CAD build for the part. Positions are in the model's coordinates, mm. Coordinates: 2 decimals unless noted, no trailing zeros. Write each loop counter-clockwise with the first axis right and the second up, starting at its lowest first coordinate (ties: lowest second). Pieces come first, ordered by that corner, then holes. Notation, with made-up numbers: M 41.5,53.25 L 81.5,53.25 A32 cw 81.5,80.25 Z; hole C 44,38 d11. An arc over 180 degrees is marked long. Put each result on its own line as item: value. Start each with the question number.
```python
from build123d import *

# Parameters (mm, degrees)
SKETCH1_R           = 76
SKETCH1_R_2         = 27.051
SKETCH1_R_3         = 2
BOSS_EXTRUDE1_DEPTH = 7
SKETCH4_R           = 6.25
CUT_EXTRUDE1_DEPTH  = 10
FILLET1_R           = 5


with BuildPart() as part:
    # Sketch1 → Boss-Extrude1 (new body)
    with BuildSketch(Plane(origin=(0, 0, 0), x_dir=(1, 0, 0), z_dir=(0, 1, 0))):
        with Locations(Location((0, 0, 0), (0, 0, 270))):
            Circle(SKETCH1_R)
        with Locations(Location((0, 0, 0), (0, 0, 270))):
            Circle(SKETCH1_R_2, mode=Mode.SUBTRACT)
        with Locations(Location((0, 62.5, 0), (0, 0, 270))):
            Circle(SKETCH1_R_3, mode=Mode.SUBTRACT)
        with Locations(Location((62.5, 0, 0), (0, 0, 270))):
            Circle(SKETCH1_R_3, mode=Mode.SUBTRACT)
        with Locations(Location((0, -62.5, 0), (0, 0, 270))):
            Circle(SKETCH1_R_3, mode=Mode.SUBTRACT)
        with Locations(Location((-62.5, 0, 0), (0, 0, 270))):
            Circle(SKETCH1_R_3, mode=Mode.SUBTRACT)
    extrude(amount=BOSS_EXTRUDE1_DEPTH)

    # Sketch4 → Cut-Extrude1 (cut)
    with BuildSketch(Plane(origin=(0, 7, 0), x_dir=(1, 0, 0), z_dir=(0, 1, 0))):
        with BuildLine():
            Line((27.751246841, -43.661149418), (17.007161012, -32.917063589))
            ThreePointArc((17.007161012, -32.917063589), (15.274204293, -33.756114768), (13.5, -34.504008477))
            Line((13.5, -34.504008477), (13.5, -62.5))
            ThreePointArc((13.5, -62.5), (25.524772494, -58.625813335), (36.553123822, -52.463026398))
            Line((36.553123822, -52.463026398), (27.751246841, -43.661149418))
        make_face()
        with BuildLine():
            Line((62.5, -13.5), (34.504008477, -13.5))
            ThreePointArc((34.504008477, -13.5), (33.756114768, -15.274204293), (32.917063589, -17.007161012))
            Line((32.917063589, -17.007161012), (43.66114941, -27.751246833))
            Line((43.66114941, -27.751246833), (52.463026398, -36.553123822))
            ThreePointArc((52.463026398, -36.553123822), (58.625813335, -25.524772494), (62.5, -13.5))
        make_face()
        with BuildLine():
            ThreePointArc((-13.5, -34.504008477), (-15.274204293, -33.756114768), (-17.007161012, -32.917063589))
            Line((-17.007161012, -32.917063589), (-27.751246874, -43.66114945))
            Line((-27.751246874, -43.66114945), (-36.553123822, -52.463026398))
            ThreePointArc((-36.553123822, -52.463026398), (-25.524772494, -58.625813335), (-13.5, -62.5))
            Line((-13.5, -62.5), (-13.5, -34.504008477))
        make_face()
        with BuildLine():
            ThreePointArc((-32.917063589, -17.007161012), (-33.756114768, -15.274204293), (-34.504008477, -13.5))
            Line((-34.504008477, -13.5), (-62.5, -13.5))
            ThreePointArc((-62.5, -13.5), (-58.625813335, -25.524772494), (-52.463026398, -36.553123822))
            Line((-52.463026398, -36.553123822), (-43.661149471, -27.751246894))
            Line((-43.661149471, -27.751246894), (-32.917063589, -17.007161012))
        make_face()
        with BuildLine():
            ThreePointArc((-34.504008477, 13.5), (-33.756114768, 15.274204293), (-32.917063589, 17.007161012))
            Line((-32.917063589, 17.007161012), (-43.66114943, 27.751246854))
            Line((-43.66114943, 27.751246854), (-52.463026398, 36.553123822))
            ThreePointArc((-52.463026398, 36.553123822), (-58.625813335, 25.524772494), (-62.5, 13.5))
            Line((-62.5, 13.5), (-34.504008477, 13.5))
        make_face()
        with BuildLine():
            ThreePointArc((-17.007161012, 32.917063589), (-15.274204293, 33.756114768), (-13.5, 34.504008477))
            Line((-13.5, 34.504008477), (-13.5, 62.5))
            ThreePointArc((-13.5, 62.5), (-25.524772494, 58.625813335), (-36.553123822, 52.463026398))
            Line((-36.553123822, 52.463026398), (-27.751246874, 43.66114945))
            Line((-27.751246874, 43.66114945), (-17.007161012, 32.917063589))
        make_face()
        with BuildLine():
            ThreePointArc((36.553123822, 52.463026398), (25.524772494, 58.625813335), (13.5, 62.5))
            Line((13.5, 62.5), (13.5, 34.504008477))
            ThreePointArc((13.5, 34.504008477), (15.274204293, 33.756114768), (17.007161012, 32.917063589))
            Line((17.007161012, 32.917063589), (27.751246906, 43.661149483))
            Line((27.751246906, 43.661149483), (36.553123822, 52.463026398))
        make_face()
        with BuildLine():
            ThreePointArc((62.5, 13.5), (58.625813335, 25.524772494), (52.463026398, 36.553123822))
            Line((52.463026398, 36.553123822), (43.66114945, 27.751246874))
            Line((43.66114945, 27.751246874), (32.917063589, 17.007161012))
            ThreePointArc((32.917063589, 17.007161012), (33.756114768, 15.274204293), (34.504008477, 13.5))
            Line((34.504008477, 13.5), (62.5, 13.5))
        make_face()
        with Locations(Location((35.706198162, 35.706198162, 0), (0, 0, 270))):
            Circle(SKETCH4_R)
        with Locations(Location((35.706198162, -35.706198162, 0), (0, 0, 270))):
            Circle(SKETCH4_R)
        with Locations(Location((-35.706198162, -35.706198162, 0), (0, 0, 270))):
            Circle(SKETCH4_R)
        with Locations(Location((-35.706198162, 35.706198162, 0), (0, 0, 270))):
            Circle(SKETCH4_R)
    extrude(amount=-CUT_EXTRUDE1_DEPTH, mode=Mode.SUBTRACT)

    # Fillet1
    # the kernel refuses this fillet: 5 mm, written as the material it adds along each edge
    with BuildSketch(Plane(origin=(34.504008477, 7, 13.5), x_dir=(1, 0, 0), z_dir=(0, -1, 0)), Plane(origin=(13.5, 7, -34.504008477), x_dir=(0, 0, -1), z_dir=(0, -1, 0)), Plane(origin=(-34.504008477, 7, -13.5), x_dir=(-1, 0, 0), z_dir=(0, -1, 0)), Plane(origin=(-13.5, 7, 34.504008477), x_dir=(0, 0, 1), z_dir=(0, -1, 0))) as fillet1_piece_1:
        with BuildLine():
            CenterArc((3.258891319, 5), FILLET1_R, 206.100178987, 63.899821013)
            ThreePointArc((-1.231239688, 2.800290124), (-0.586707725, 1.412857227), (0, 0))
            Line((0, 0), (3.258891319, 0))
        make_face()
    extrude(amount=7)
    with BuildSketch(Plane(origin=(62.5, 7, 13.5), x_dir=(-1, 0, 0), z_dir=(0, -1, 0))) as fillet1_piece_2:
        with BuildLine():
            CenterArc((6.537189081, -5), FILLET1_R, 90, 108.2926811)
            ThreePointArc((1.789861186, -6.569355874), (0.807426008, -3.308519097), (0, 0))
            Line((0, 0), (6.537189081, 0))
        make_face()
    extrude(amount=7)
    with BuildSketch(Plane(origin=(52.463026398, 7, 36.553123822), x_dir=(-0.7071067811865521, 0, -0.707106781186543), z_dir=(0, -1, 0)), Plane(origin=(-36.553123822, 7, 52.463026398), x_dir=(0.7071067811865515, 0, -0.7071067811865436), z_dir=(0, -1, 0))) as fillet1_piece_3:
        with BuildLine():
            CenterArc((6.286852353, 5), FILLET1_R, 163.996405934, 106.003594066)
            ThreePointArc((1.480630334, 6.378488268), (0.658610883, 3.208210045), (0, 0))
            Line((0, 0), (6.286852353, 0))
        make_face()
    extrude(amount=7)
    with BuildSketch(Plane(origin=(32.917063589, 7, 17.007161012), x_dir=(0.4193809358930841, 0, -0.907810349472532), z_dir=(0, -1, 0)), Plane(origin=(17.007161012, 7, -32.917063589), x_dir=(-0.9078103494725283, 0, -0.41938093589309267), z_dir=(0, -1, 0)), Plane(origin=(-32.917063589, 7, -17.007161012), x_dir=(-0.4193809358930852, 0, 0.9078103494725317), z_dir=(0, -1, 0))) as fillet1_piece_4:
        with BuildLine():
            CenterArc((3.489548398, 4.995132399), FILLET1_R, 200.204490443, 67.267112024)
            Line((-1.202781391, 3.268273647), (0, 0))
            ThreePointArc((0, 0), (1.634487847, 0.036069898), (3.268975694, 0))
        make_face()
    extrude(amount=7)
    with BuildSketch(Plane(origin=(32.917063589, 7, -17.007161012), x_dir=(0.7071067811865526, 0, -0.7071067811865425), z_dir=(0, -1, 0)), Plane(origin=(-17.007161012, 7, -32.917063589), x_dir=(-0.7071067811865506, 0, -0.7071067811865445), z_dir=(0, -1, 0)), Plane(origin=(-32.917063589, 7, 17.007161012), x_dir=(-0.7071067811865506, 0, 0.7071067811865445), z_dir=(0, -1, 0)), Plane(origin=(17.007161012, 7, 32.917063589), x_dir=(0.7071067811865501, 0, 0.707106781186545), z_dir=(0, -1, 0))) as fillet1_piece_5:
        with BuildLine():
            CenterArc((3.482570273, 5), FILLET1_R, 202.732887976, 67.267112024)
            ThreePointArc((-1.129011858, 3.067822406), (-0.530655558, 1.546368727), (0, 0))
            Line((0, 0), (3.482570273, 0))
        make_face()
    extrude(amount=7)
    with BuildSketch(Plane(origin=(34.504008477, 7, -13.5), x_dir=(1, 0, 0), z_dir=(0, -1, 0))) as fillet1_piece_6:
        with BuildLine():
            CenterArc((3.258891319, -5), FILLET1_R, 90, 63.899821013)
            ThreePointArc((-1.231239688, -2.800290124), (-0.586707725, -1.412857227), (0, 0))
            Line((0, 0), (3.258891319, 0))
        make_face()
    extrude(amount=7)
    with BuildSketch(Plane(origin=(62.5, 7, -13.5), x_dir=(-1, 0, 0), z_dir=(0, -1, 0)), Plane(origin=(-13.5, 7, -62.5), x_dir=(0, 0, 1), z_dir=(0, -1, 0)), Plane(origin=(-62.5, 7, 13.5), x_dir=(1, 0, 0), z_dir=(0, -1, 0)), Plane(origin=(13.5, 7, 62.5), x_dir=(0, 0, -1), z_dir=(0, -1, 0))) as fillet1_piece_7:
        with BuildLine():
            CenterArc((6.537189081, 5), FILLET1_R, 161.7073189, 108.2926811)
            ThreePointArc((1.789861186, 6.569355874), (0.807426008, 3.308519097), (0, 0))
            Line((0, 0), (6.537189081, 0))
        make_face()
    extrude(amount=7)
    with BuildSketch(Plane(origin=(52.463026398, 7, -36.553123822), x_dir=(0.5289042688396526, 0, 0.848681491728901), z_dir=(0, -1, 0))) as fillet1_piece_8:
        with BuildLine():
            CenterArc((6.292063112, 4.993441128), FILLET1_R, 166.931450544, 106.003594066)
            Line((1.421561948, 6.124024341), (0, 0))
            ThreePointArc((0, 0), (3.274041034, -0.08387667), (6.548082068, 0))
        make_face()
    extrude(amount=7)
    with BuildSketch(Plane(origin=(36.553123822, 7, -52.463026398), x_dir=(-0.8486814917288963, 0, -0.52890426883966), z_dir=(0, -1, 0)), Plane(origin=(-52.463026398, 7, -36.553123822), x_dir=(-0.5289042688396536, 0, 0.8486814917289003), z_dir=(0, -1, 0))) as fillet1_piece_9:
        with BuildLine():
            CenterArc((6.292063112, -4.993441128), FILLET1_R, 87.06495539, 106.003594066)
            Line((1.421561948, -6.124024341), (0, 0))
            ThreePointArc((0, 0), (3.274041034, 0.08387667), (6.548082068, 0))
        make_face()
    extrude(amount=7)
    with BuildSketch(Plane(origin=(13.5, 7, -62.5), x_dir=(0.9648302017860143, 0, 0.26287388938720957), z_dir=(0, -1, 0)), Plane(origin=(-62.5, 7, -13.5), x_dir=(0.2628738893872084, 0, -0.9648302017860146), z_dir=(0, -1, 0)), Plane(origin=(-13.5, 7, 62.5), x_dir=(-0.9648302017860145, 0, -0.26287388938720885), z_dir=(0, -1, 0))) as fillet1_piece_10:
        with BuildLine():
            CenterArc((6.542607328, 4.992908013), FILLET1_R, 164.759342849, 108.2926811)
            Line((1.718456319, 6.30727746), (0, 0))
            ThreePointArc((0, 0), (3.404410363, -0.090694285), (6.808820725, 0))
        make_face()
    extrude(amount=7)
    with BuildSketch(Plane(origin=(-36.553123822, 7, -52.463026398), x_dir=(0.707106781186552, 0, 0.7071067811865429), z_dir=(0, -1, 0)), Plane(origin=(-52.463026398, 7, 36.553123822), x_dir=(0.7071067811865515, 0, -0.7071067811865436), z_dir=(0, -1, 0)), Plane(origin=(36.553123822, 7, 52.463026398), x_dir=(-0.7071067811865527, 0, -0.7071067811865425), z_dir=(0, -1, 0))) as fillet1_piece_11:
        with BuildLine():
            CenterArc((6.286852353, -5), FILLET1_R, 90, 106.003594066)
            ThreePointArc((1.480630334, -6.378488268), (0.658610883, -3.208210045), (0, 0))
            Line((0, 0), (6.286852353, 0))
        make_face()
    extrude(amount=7)
    with BuildSketch(Plane(origin=(-13.5, 7, -34.504008477), x_dir=(-0.9154220062230544, 0, 0.4024954043496127), z_dir=(0, -1, 0)), Plane(origin=(-34.504008477, 7, 13.5), x_dir=(0.4024954043496181, 0, 0.915422006223052), z_dir=(0, -1, 0)), Plane(origin=(13.5, 7, 34.504008477), x_dir=(0.915422006223051, 0, -0.40249540434962), z_dir=(0, -1, 0))) as fillet1_piece_12:
        with BuildLine():
            CenterArc((3.265421252, 4.995737851), FILLET1_R, 203.734271223, 63.899821013)
            Line((-1.311688779, 2.983260829), (0, 0))
            ThreePointArc((0, 0), (1.52950776, 0.031583378), (3.059015519, 0))
        make_face()
    extrude(amount=7)
    with BuildSketch(Plane(origin=(-17.007161012, 7, 32.917063589), x_dir=(-0.7071067811865496, 0, 0.7071067811865455), z_dir=(0, -1, 0))) as fillet1_piece_13:
        with BuildLine():
            CenterArc((3.482570273, -5), FILLET1_R, 90, 67.267112024)
            ThreePointArc((-1.129011858, -3.067822406), (-0.530655558, -1.546368727), (0, 0))
            Line((0, 0), (3.482570273, 0))
        make_face()
    extrude(amount=7)


solid = part.part
```
(1) Two-plate mould, pull along Z, no slides. Class faces 1 (the face through (33.514, 3.549, -52.313)), 2 (the face through (22, 7, -24)), 3 (the face through (34.165, 3.549, -17.496)): +Z half, -Z half, draft (parallel to the pull), parting line (faces both ways), or undercut.
(2) Drill centre lines: line 1 (X direction, y = 3, z = 0); line 2 (X direction, y = 5.5, z = 22.5); line 3 (Z direction, x = 15.5, y = 3.75). Where is each one in solid material? Low to high. Write a range as [from, to].
(3) Drop flat-ended pins along their axis: pin 1 (7.5 mm diameter, centred on x = 35.71, z = -35.71, fed in from -Y); pin 2 (4 mm diameter, centred on y = 2.5, z = 11.5, fed in from +X); pin 3 (3 mm diameter, centred on x = 55.5, y = 4, fed in from -Z); pin 4 (1.5 mm diameter, centred on x = 57, y = 4.5, fed in from -Z). Give the stop position or say it passes through.
(4) Slice it at D-D, the plane y = 5. State how many separate pieces and enclosed holes the cut face has, then the cut area to 3 significant figures.
(5) Slice it at A-A, the plane x = 0. Write the cut outline in (y, z), then the cut area to 3 significant figures.
(6) Slice it at C-C, the plane z = -52.5. Write the cut outline in (x, y), then the cut area to 3 significant figures.
(7) Slice it at B-B, the plane z = 0. Write the cut outline in (x, y), then the cut area to 3 significant figures.
Result set:
1. face 1: undercut
1. face 2: draft
1. face 3: undercut
2. line 1: x = [-76, -64.5], [-60.5, -27.05], [27.05, 60.5], [64.5, 76]
2. line 2: x = [-72.59, -59.85], [-38.41, -15.02], [15.02, 38.41], [59.85, 72.59]
2. line 3: z = [-74.4, -59.96], [-33.93, -22.17], [22.17, 33.93], [59.96, 74.4]
3. pin 1: passes through
3. pin 2: stops at x = 75.4
3. pin 3: stops at z = -53.48
3. pin 4: stops at z = -51.11
4. separate pieces: 1
4. enclosed holes: 17
4. area: 12,300 mm^2
5. outline: M 0,-76 L 7,-76 L 7,-64.5 L 0,-64.5 Z; M 0,-60.5 L 7,-60.5 L 7,-27.05 L 0,-27.05 Z; M 0,27.05 L 7,27.05 L 7,60.5 L 0,60.5 Z; M 0,64.5 L 7,64.5 L 7,76 L 0,76 Z
5. area: 629 mm^2
6. outline: M -54.95,0 L -33.48,0 L -33.48,7 L -54.95,7 Z; M -13.5,0 L 13.5,0 L 13.5,7 L -13.5,7 Z; M 33.48,0 L 54.95,0 L 54.95,7 L 33.48,7 Z
6. area: 490 mm^2
7. outline: M -76,0 L -64.5,0 L -64.5,7 L -76,7 Z; M -60.5,0 L -27.05,0 L -27.05,7 L -60.5,7 Z; M 27.05,0 L 60.5,0 L 60.5,7 L 27.05,7 Z; M 64.5,0 L 76,0 L 76,7 L 64.5,7 Z
7. area: 629 mm^2
